Solid Edge part; units mm, degrees
sketch "Sketch1" plane through (0, 0, 0) normal (0, -1, 0) x (1, 0, 0)
  line L0 (4, 12) -> (4, 0)
  line L1 (4, 0) -> (11, 0)
  line L2 (11, 0) -> (11, 2)
  line L3 (11, 2) -> (5, 2)
  line L4 (5, 2) -> (5, 12)
  line L5 (5, 12) -> (4, 12)
  dimension "D1" = 4
  dimension "D2" = 11
revolve "RevolvedProtrusion1" add sketch "Sketch1" angle 360 about axis through (0, 0, 54) along (0, 0, -1)
hole "Hole1" at (8, 0, 2) direction (0, 0, -1) diameter 3.6 end up to next
pattern_circular "Pattern1" count 4 over 360 about axis through (0, 0, 2) along (0, 0, 1) of "Hole1"
chamfer "Chamfer_1" distance 0.5 angle 30 2 edges at (-4, 0, 12) (-4, 0, 0) measured on face at (2.2136, -3.3317, 9.88)
properties material "Stainless steel"
For this review, take the finished solid that the model builds, in its own axes (mm). A direction names the side the tool comes from. Round coordinates to 2 decimals unless told otherwise and drop trailing zeros. Loops run counter-clockwise (first coordinate to the right, second up) from the corner with the lowest first, then second, coordinate; pieces in that order, holes last. Notation, with made-up numbers: (60, 36.5) - (88, 36.5) arc R19 ccw to (88, 61.5) - close; hole circle Ø11 at (66.25, -29). An arc over 180 degrees is marked (long way). Use one line per item in the form item = value.
1) Clearance check with flat-ended pins moving along their axes: P1, Ø4.5, axis at x = -8, y = 0, coming from the -Z side; P2, Ø3, axis at x = 0, y = 8, coming from the +Z side; P3, Ø2, axis at x = -5, z = 6.5, coming from the -Y side; P4, Ø4, axis at y = 4, z = 3.5, coming from the +X side. State where each tip first meets the part, or that it passes through.
Solutions:
P1 = 0
P2 = through
P3 = -3
P4 = 10.67
2) Tool access review of faces 1 (the face through (0.39, -6.243, 1.014)), 2 (the face through (5, 2, 2)): name each direction out of +Z, -Z, +X, -X, +Y, -Y from which nothing blocks a thin tool from reaching the whole face with its end or side.
Solutions:
face_1 = +Z, -Z
face_2 = +Z
3) Mouldability with a two-part tool opening along X and no side actions: class faces 3 (the face through (2, -4, 12)), 4 (the face through (-1.08, -4.88, 7.07)), 5 (the face through (-0.39, 6.243, 1.014)) as pulls with the +X half, pulls with the -X half, needs draft (parallel to the pull), parting line crosses it, or undercut.
Solutions:
face_3 = needs draft
face_4 = parting line crosses it
face_5 = undercut
4) We need section C-C on z = 1.25. Write out the cut boundary in (x, y), then the cut area to 3 significant figures.
Solutions:
outline = circle Ø22 at (0, 0); hole circle Ø3.6 at (-8, 0); hole circle Ø8 at (0, 0); hole circle Ø3.6 at (0, -8); hole circle Ø3.6 at (0, 8); hole circle Ø3.6 at (8, 0)
area = 289 mm2
5) We need section A-A on x = 0. Write out the cut boundary in (y, z).
Solutions:
outline = (-11, 0) - (-9.8, 0) - (-9.8, 2) - (-11, 2) - close; (-6.2, 0) - (-4.29, 0) - (-4, 0.5) - (-4, 11.5) - (-4.29, 12) - (-5, 12) - (-5, 2) - (-6.2, 2) - close; (4, 0.5) - (4.29, 0) - (6.2, 0) - (6.2, 2) - (5, 2) - (5, 12) - (4.29, 12) - (4, 11.5) - close; (9.8, 0) - (11, 0) - (11, 2) - (9.8, 2) - close
6) We need section D-D on y = -8.5. Write out the cut boundary in (x, z), then the cut area to 3 significant figures.
Solutions:
outline = (-6.98, 0) - (-1.73, 0) - (-1.73, 2) - (-6.98, 2) - close; (1.73, 0) - (6.98, 0) - (6.98, 2) - (1.73, 2) - close
area = 21.0 mm2
7) Wall thickness on probe 1 along X at (y, z) = (0, 1.4); probe 2 along Z at (x, y) = (5.75, 5): over which ranges is each line inside the solid? List them lowest first.
Solutions:
probe_1 = -11 to -9.8, -6.2 to -4, 4 to 6.2, 9.8 to 11
probe_2 = 0 to 2
